from build123d import *

# Parameters (mm, degrees)
SKETCH1_W           = 80
SKETCH1_H           = 300
SKETCH1_R           = 12.4
SKETCH1_R_2         = 5
BOSS_EXTRUDE2_DEPTH = 25


with BuildPart() as part:
    # Sketch1 → Boss-Extrude2 (new body)
    with BuildSketch(Plane.XY):
        with Locations((-40, 150)):
            Rectangle(SKETCH1_W, SKETCH1_H)
        with Locations((-40, 200)):
            Circle(SKETCH1_R, mode=Mode.SUBTRACT)
        with Locations((-40, 35)):
            Circle(SKETCH1_R_2, mode=Mode.SUBTRACT)
        with Locations((-40, 100)):
            Circle(SKETCH1_R_2, mode=Mode.SUBTRACT)
    extrude(amount=-BOSS_EXTRUDE2_DEPTH)


solid = part.part
Here's how the part is built. I have some questions about the finished solid (model axes, mm). Round coordinates to 2 decimals unless told otherwise and drop trailing zeros. Loops run counter-clockwise (first coordinate to the right, second up) from the corner with the lowest first, then second, coordinate; pieces in that order, holes last. Notation, with made-up numbers: M 61.25,19.25 L 110.25,19.25 A15 ccw 110.25,34.25 Z; hole C -2.5,-1.5 d6. An arc over 180 degrees is marked long. Write each question's results on one line, items separated by ' | '. Start each with the question number.
(1) I want a section at B-B (x = -40). Please give me the cut outline in (y, z).
(2) I want a section at A-A (y = 100). Please give me the cut outline in (x, z).
(3) If I drill on probe 1 along Y at (x, z) = (-40, -8.25); probe 2 along X at (y, z) = (209, -11.5); probe 3 along X at (y, z) = (31, -14.25), over which ranges is the centre line in solid material (lowest first)? Write a range as from..to.
(4) I want a section at C-C (z = -7.5). Please give me the cut outline in (x, y).
(5) Thinking about a two-plate mould opening in X: for faces 1 (the flat face through (0, 148, -12)), 2 (the cylindrical face through (-45, 100, -12)), 3 (the flat face through (-80, 148, -12)), which applies, pulls with the +X half, pulls with the -X half, needs draft (parallel to the pull), parting line crosses it, or undercut?
(6) I want a section at D-D (y = 200). Please give me the cut outline in (x, z).
Solved:
1) outline: M 0,-25 L 30,-25 L 30,0 L 0,0 Z; M 40,-25 L 95,-25 L 95,0 L 40,0 Z; M 105,-25 L 187.6,-25 L 187.6,0 L 105,0 Z; M 212.4,-25 L 300,-25 L 300,0 L 212.4,0 Z
2) outline: M -80,-25 L -45,-25 L -45,0 L -80,0 Z; M -35,-25 L 0,-25 L 0,0 L -35,0 Z
3) probe 1: y = 0..30, 40..95, 105..187.6, 212.4..300 | probe 2: x = -80..-48.53, -31.47..0 | probe 3: x = -80..-43, -37..0
4) outline: M -80,0 L 0,0 L 0,300 L -80,300 Z; hole C -40,200 d24.8; hole C -40,35 d10; hole C -40,100 d10
5) face 1: pulls with the +X half | face 2: undercut | face 3: pulls with the -X half
6) outline: M -80,-25 L -52.4,-25 L -52.4,0 L -80,0 Z; M -27.6,-25 L 0,-25 L 0,0 L -27.6,0 Z
